Part model, mm, in its own coordinate system. Coordinates: 2 decimals unless noted, no trailing zeros. Loops run counter-clockwise (first coordinate to the right, second up) from the corner with the lowest first, then second, coordinate; pieces in that order, holes last. Notation, with made-up numbers: (82, 74) - (111, 74) arc R22 cw to (111, 113) - close; hole circle Ø5 at (83.25, -38.75). An arc over 180 degrees is marked (long way). One line per question, with ' | ' between items. Start each with the question number.
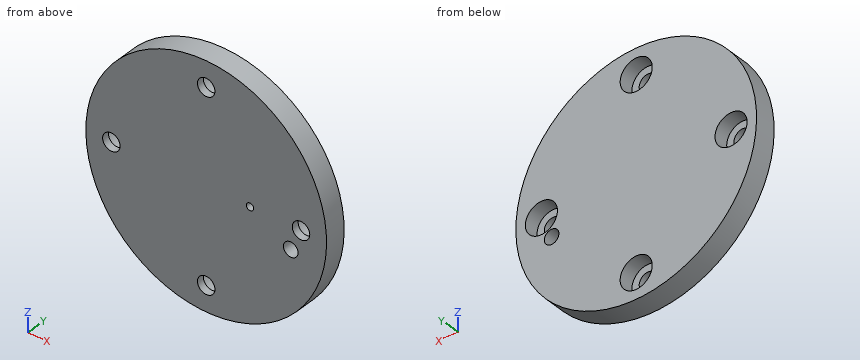
from build123d import *

# Parameters (mm, degrees)
SKETCH1_R                      = 16.5
BOSS_EXTRUDE1_DEPTH            = 3
CBORE_FOR_M2_SHCS1_D           = 2.4
CBORE_FOR_M2_SHCS1_CBORE_D     = 4.4
CBORE_FOR_M2_SHCS1_CBORE_DEPTH = 2
CIRPATTERN1_COUNT              = 4
SKETCH15_R                     = 0.5
CUT_EXTRUDE1_DEPTH             = 1.5
CUT_EXTRUDE2_DEPTH             = 24.526580712
CUT_EXTRUDE2_DEPTH_BACK        = 24.526580712
SKETCH16_R                     = 1


with BuildPart() as part:
    # Sketch1 → Boss-Extrude1 (new body)
    with BuildSketch(Plane(origin=(0, 0, 0), x_dir=(1, 0, 0), z_dir=(0, 1, 0))):
        with Locations(Location((0, 0, 0), (0, 0, 270))):
            Circle(SKETCH1_R)
    extrude(amount=BOSS_EXTRUDE1_DEPTH)

    # CBORE for M2 SHCS1 (through all)
    with Locations(Plane(origin=(0, 3, 0), x_dir=(1, 0, 0), z_dir=(0, 1, 0))):
        with Locations((-13, 0)):
            cbore_for_m2_shcs1 = CounterBoreHole(CBORE_FOR_M2_SHCS1_D / 2, CBORE_FOR_M2_SHCS1_CBORE_D / 2, CBORE_FOR_M2_SHCS1_CBORE_DEPTH)

    # CirPattern1: CBORE for M2 SHCS1 ×4 about axis
    cirpattern1_axis = Axis((0, 0, 0), (0, 1, 0))
    for i in range(1, CIRPATTERN1_COUNT):
        add(cbore_for_m2_shcs1.rotate(cirpattern1_axis, i * 360 / CIRPATTERN1_COUNT), mode=Mode.SUBTRACT)

    # Sketch15 → Cut-Extrude1 (cut)
    with BuildSketch(Plane.XZ):
        with Locations(Location((6, 0, 0), (0, 0, 270))):
            Circle(SKETCH15_R)
    extrude(amount=-CUT_EXTRUDE1_DEPTH, mode=Mode.SUBTRACT)

    # Sketch16 → Cut-Extrude2 (cut, two sides: drawn at the far end of the back side and taken through both)
    with BuildSketch(Plane(origin=(0, 3, 0), x_dir=(1, 0, 0), z_dir=(0, 1, 0)).offset(-CUT_EXTRUDE2_DEPTH_BACK)):
        with Locations(Location((11.591109915, 3.105828541, 0), (0, 0, 270))):
            Circle(SKETCH16_R)
    extrude(amount=CUT_EXTRUDE2_DEPTH + CUT_EXTRUDE2_DEPTH_BACK, mode=Mode.SUBTRACT)


solid = part.part
1) Band-saw the part on B-B on z = 0. List the corners of the cut face in (x, y).
2) Band-saw the part on D-D on x = 13. List the corners of the cut face in (y, z), then the cut area to 3 significant figures.
3) Wall check: line 1 along Z through (x, y) = (1, 0.6); line 2 along X through (y, z) = (1.6, 13). Give the ranges that are in metal, low to high. Write a range as [from, to].
4) Band-saw the part on C-C on y = 2.5. List the corners of the cut face in (x, z).
5) Band-saw the part on A-A on x = 0. List the corners of the cut face in (y, z).
6) Pin check, flat tips, straight feed: pin 1 Ø0.5 at (x, z) = (6, 0) entering from -Y; pin 2 Ø1 at (y, z) = (1.5, -3.5) entering from +X (3 decimals); pin 3 Ø1 at (x, y) = (-9, 0.5) entering from -Z; pin 4 Ø1.4 at (x, z) = (0, -13) entering from -Y. Stop position of each tip, or through.
Values found:
1) outline: (-16.5, 0) - (-14.2, 0) - (-14.2, 1) - (-15.2, 1) - (-15.2, 3) - (-16.5, 3) - close; (-11.8, 0) - (5.5, 0) - (5.5, 1.5) - (6.5, 1.5) - (6.5, 0) - (11.8, 0) - (11.8, 1) - (10.8, 1) - (10.8, 3) - (-10.8, 3) - (-10.8, 1) - (-11.8, 1) - close; (14.2, 0) - (16.5, 0) - (16.5, 3) - (15.2, 3) - (15.2, 1) - (14.2, 1) - close
2) outline: (0, -10.16) - (3, -10.16) - (3, -2.2) - (1, -2.2) - (1, -1.2) - (0, -1.2) - close; (0, 1.2) - (1, 1.2) - (1, 2.2) - (3, 2.2) - (3, 10.16) - (0, 10.16) - close | area: 49.8 mm²
3) line 1: [-16.47, -13.66], [-12.34, 12.34], [13.66, 16.47] | line 2: [-10.16, -2.2], [2.2, 10.16]
4) outline: circle Ø33 at (0, 0); hole circle Ø4.4 at (-13, 0); hole circle Ø4.4 at (0, -13); hole circle Ø4.4 at (0, 13); hole circle Ø2 at (11.59, -3.11); hole circle Ø4.4 at (13, 0)
5) outline: (0, -16.5) - (3, -16.5) - (3, -15.2) - (1, -15.2) - (1, -14.2) - (0, -14.2) - close; (0, -11.8) - (1, -11.8) - (1, -10.8) - (3, -10.8) - (3, 10.8) - (1, 10.8) - (1, 11.8) - (0, 11.8) - close; (0, 14.2) - (1, 14.2) - (1, 15.2) - (3, 15.2) - (3, 16.5) - (0, 16.5) - close
6) pin 1: y = 1.5 | pin 2: x = 16.225 | pin 3: z = -14.14 | pin 4: through
